Verification items for the finished model (mm, model axes). Coordinates: 2 decimals unless noted, no trailing zeros. Write each loop counter-clockwise with the first axis right and the second up, starting at its lowest first coordinate (ties: lowest second). Pieces come first, ordered by that corner, then holes. Notation, with made-up numbers: M 76.25,54.25 L 86.25,54.25 A25 ccw 86.25,80.25 Z; hole C 66.25,70 d1. An arc over 180 degrees is marked long. One line per item, written item: value.
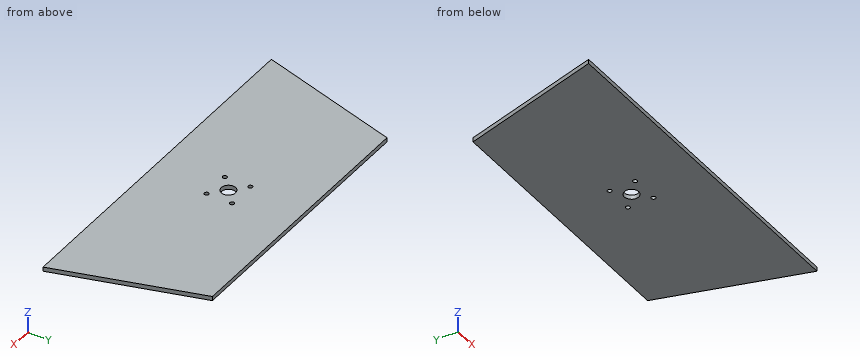
```python
from build123d import *

# Parameters (mm, degrees)
BOSS_EXTRUDE1_DEPTH        = 3
BOSS_EXTRUDE1_DEPTH_BACK   = 0.006725904
F_10_0MM_DOWEL_HOLE1_D     = 10
F_10_0MM_DOWEL_HOLE1_DEPTH = 3.006725904
F_3_0MM_DOWEL_HOLE1_D      = 3
F_3_0MM_DOWEL_HOLE1_DEPTH  = 3.006725904


with BuildPart() as part:
    # Sketch1 → Boss-Extrude1 (new body, two sides)
    with BuildSketch(Plane.XY) as boss_extrude1_sk:
        Polygon((-3.5, 0), (245, 0), (215.720058283, 100), (25.779941717, 100), align=None)
    extrude(amount=BOSS_EXTRUDE1_DEPTH)
    extrude(boss_extrude1_sk.sketch, amount=-BOSS_EXTRUDE1_DEPTH_BACK)

    # Ø10.0mm Dowel Hole1
    with Locations(Plane.XY.offset(3)):
        with Locations((120.75, 50)):
            Hole(F_10_0MM_DOWEL_HOLE1_D / 2, depth=F_10_0MM_DOWEL_HOLE1_DEPTH)

    # Ø3.0mm Dowel Hole1
    with Locations(Plane.XY.offset(3)):
        with Locations((110.8, 58.95), (130.7, 58.95), (130.7, 41.05), (110.8, 41.05)):
            Hole(F_3_0MM_DOWEL_HOLE1_D / 2, depth=F_3_0MM_DOWEL_HOLE1_DEPTH)


solid = part.part
```
Item 1: Scan lines: line 1 (Y direction, x = 111, z = 1.65); line 2 (Y direction, x = 120.75, z = 1.6); line 3 (X direction, y = 65.5, z = 1.85). Record each from-to range of solid material in increasing order.
The answers:
line 1: y = 0 to 39.56, 42.54 to 57.46, 60.44 to 100
line 2: y = 0 to 45, 55 to 100
line 3: x = 15.68 to 225.82
Item 2: Cross-section at A-A, the plane x = 120.75. Enter the section's corners in (y, z).
The answers:
outline: M 0,-0.01 L 45,-0.01 L 45,3 L 0,3 Z; M 55,-0.01 L 100,-0.01 L 100,3 L 55,3 Z
Item 3: Cross-section at B-B, the plane z = 0.6. Enter the section's corners in (x, y).
The answers:
outline: M -3.5,0 L 245,0 L 215.72,100 L 25.78,100 Z; hole C 110.8,41.05 d3; hole C 110.8,58.95 d3; hole C 120.75,50 d10; hole C 130.7,41.05 d3; hole C 130.7,58.95 d3
Item 4: Cross-section at D-D, the plane y = 71. Enter the section's corners in (x, z), and give its area (3 significant figures).
The answers:
outline: M 17.29,-0.01 L 224.21,-0.01 L 224.21,3 L 17.29,3 Z
area: 622 mm²
Item 5: Cross-section at C-C, the plane y = 50. Enter the section's corners in (x, z), and give its area (3 significant figures).
The answers:
outline: M 11.14,-0.01 L 115.75,-0.01 L 115.75,3 L 11.14,3 Z; M 125.75,-0.01 L 230.36,-0.01 L 230.36,3 L 125.75,3 Z
area: 629 mm²
